Geometry: final body of the model. Coordinates: model frame, mm. A direction names the side the tool comes from. Coordinates: 2 decimals unless noted, no trailing zeros. Order: outer loops, then holes, each group sorted by start corner. A loop starts at its lowest first (then second) coordinate and runs counter-clockwise, first axis right, second up. Notation, with made-up numbers: M 49,21 L 65,21 A12 ccw 65,41 Z; hole C 5.25,-37.75 d9. An arc over 180 degrees is marked long. Write item = value, one per line.
from build123d import *

# Parameters (mm, degrees)
F0_W          = 518
F0_H          = 10
F1_DEPTH      = 1474
F2_T          = -1
F3_R          = 2
F4_DEPTH      = 10
F4_DEPTH_BACK = 1490
F5_R          = 12.5
F6_DEPTH      = 5
F7_SIZE       = 3
F8_W          = 1.794569
F8_H          = 11.12199
F9_DEPTH      = 5
F10_W         = 102.76919
F10_H         = 149.015308
F11_DEPTH     = 15
F12_W         = 150
F12_H         = 1375
F13_DEPTH     = 15


with BuildPart() as f1:
    # F0 (on Top) → F1 (new body)
    with BuildSketch(Plane.XY):
        with Locations((259, 5)):
            Rectangle(F0_W, F0_H)
    extrude(amount=F1_DEPTH)

    # F2
    f2_openings = [f1.faces().sort_by_distance(p)[0] for p in [
        (259, 10, 737),
    ]]
    offset(amount=F2_T, openings=f2_openings)

    # F3 (on face) → F4 (join, two sides)
    with BuildSketch(Plane(origin=(0, 0, 0), x_dir=(1, 0, 0), z_dir=(0, 0, -1))) as f4_sk:
        with Locations((509, -5)):
            Circle(F3_R)
    extrude(amount=F4_DEPTH)
    extrude(f4_sk.sketch, amount=-F4_DEPTH_BACK)

    # F5 (on face) → F6 (join)
    with BuildSketch(Plane.XZ):
        with Locations((56.609962, 824)):
            Circle(F5_R)
    extrude(amount=F6_DEPTH)

    # F7
    f7_edges = [f1.edges().sort_by_distance(p)[0] for p in [
        (44.109962, -5, 824),
    ]]
    chamfer(f7_edges, length=F7_SIZE)

    # F8 (on face) → F9 (cut)
    with BuildSketch(Plane.XZ.offset(5)):
        with Locations((56.609962, 824)):
            Rectangle(F8_W, F8_H)
    extrude(amount=-F9_DEPTH, mode=Mode.SUBTRACT)

    # F10 (on face) → F11 (join)
    with BuildSketch(Plane(origin=(0, 1, 0), x_dir=(-1, 0, 0), z_dir=(0, 1, 0))):
        with Locations((-56.717325, 824.265957)):
            Rectangle(F10_W, F10_H)
    extrude(amount=F11_DEPTH)

    # F12 (on face) → F13 (join)
    with BuildSketch(Plane(origin=(0, 1, 0), x_dir=(-1, 0, 0), z_dir=(0, 1, 0))):
        with Locations((-259, 736.5)):
            Rectangle(F12_W, F12_H)
    extrude(amount=F13_DEPTH)


solid = f1.part
1) Set-up query: faces 4 (the face through (260, 16, 746)), 5 (the face through (53.9, -0.986, 811.797)). Return all of +Z, -Z, +X, -X, +Y, -Y with unobstructed straight access to the full face (end or side cutting, diameter ignored); none if empty.
Numbers:
face_4 = +Z, -Z, +X, -X, +Y
face_5 = -Y
2) Pin query (flat end, axial travel): pin 1 (4.5 mm diameter, centred on y = 7.5, z = 900, fed in from -X); pin 2 (1 mm diameter, centred on x = 152.5, z = 1262, fed in from +Y); pin 3 (7 mm diameter, centred on x = 135, y = 7, fed in from +Z); pin 4 (0.9 mm diameter, centred on x = 56.5, y = -2.5, fed in from +Z). Return the tip coordinate at first contact, or that it passes through.
Numbers:
pin_1 = 0
pin_2 = 1
pin_3 = 1474
pin_4 = 836.45
3) Section C-C, the plane z = 449. Return loops of the section in (x, y), and give its area (3 significant figures).
Numbers:
outline = M 0,0 L 518,0 L 518,10 L 517,10 L 517,1 L 334,1 L 334,16 L 184,16 L 184,1 L 1,1 L 1,10 L 0,10 Z; C 509,5 d4
area = 2,800 mm²
4) Section A-A, the plane z = 859.5. Return loops of the section in (x, y).
Numbers:
outline = M 0,0 L 518,0 L 518,10 L 517,10 L 517,1 L 334,1 L 334,16 L 184,16 L 184,1 L 108.1,1 L 108.1,16 L 5.33,16 L 5.33,1 L 1,1 L 1,10 L 0,10 Z; C 509,5 d4
5) Line query: L1, parallel to Z at x = 57.5, y = 1.25; L2, parallel to X at y = 8.5, z = 733.5; L3, parallel to Z at x = 239, y = 1.25. Output: solid intervals per line, ascending.
Numbers:
L1 = 0 to 1, 749.76 to 898.77, 1473 to 1474
L2 = 0 to 1, 184 to 334, 517 to 518
L3 = 0 to 1, 49 to 1424, 1473 to 1474
6) Section B-B, the plane x = 248. Return loops of the section in (y, z), and give its area (3 significant figures).
Numbers:
outline = M 0,0 L 10,0 L 10,1 L 1,1 L 1,49 L 16,49 L 16,1424 L 1,1424 L 1,1473 L 10,1473 L 10,1474 L 0,1474 Z
area = 22,100 mm²
7) Mould query, pull axis X, two halves, no side actions, for faces 1 (the face through (57, 16, 825)), 2 (the face through (65.52, -4.854, 820.306)), 3 (the face through (370, 1, 727)). Classes: pulls with the +X half, pulls with the -X half, needs draft (parallel to the pull), parting line crosses it, or undercut.
Numbers:
face_1 = needs draft
face_2 = parting line crosses it
face_3 = undercut
